For this review, take the finished solid that the model builds, in its own axes (mm). Face numbers are marked on the shaded views. A direction names the side the tool comes from. Give positions to 0.01 mm unless a question says otherwise; leave off trailing zeros. Order: outer loops, then holes, each group sorted by start corner. A loop starts at its lowest first (then second) coordinate and runs counter-clockwise, first axis right, second up.
Item 1: The part is to be moulded in two halves that separate along X. For the marked faces 4, 5 and 6, say which applies: released by +X, released by -X, zero draft, split by the parting line, or undercut.
Item 2: For probe 1 along X at (y, z) = (1.75, -10.75); probe 2 along X at (y, z) = (8.5, -14.25); probe 3 along Y at (x, z) = (-4, -9), list the stretches that pass through material, from the lowest coordinate up.
Item 3: Consider section A-A (x = 0). Give the boundary of the cut face in (y, z), plus the area to 3 significant figures.
Item 4: Consider section D-D (x = 2.5). Give the boundary of the cut face in (y, z), plus the area to 3 significant figures.
Item 5: Machinability: for the marked faces 1, 2 and 3, which of the approach directions +Z, -Z, +X, -X, +Y, -Y give a long, thin tool a straight path to every point of the face, cutting with its end or side? Answer none if there is none.
Item 6: Consider section B-B (z = -11). Give the boundary of the cut face in (x, y), plus the area to 3 significant figures.
Item 7: For P1, Ø6, axis at y = 16, z = -10.5, coming from the -X side; P2, Ø1, axis at x = 4, z = -17.5, coming from the +Y side, all flat-tipped, find the tip position at first contact; note any pin that passes through.
Item 8: Consider section C-C (y = 12). Give the boundary of the cut face in (x, z), plus the area to 3 significant figures.
```python
from build123d import *

# Parameters (mm, degrees)
BODY_DEPTH     = 8.5
SKETCH2_W      = 13
SKETCH2_H      = 17
EXTUSION_DEPTH = 18
HOLE_A_DEPTH   = 29.217902119
HOLE_B_DEPTH   = 17


with BuildPart() as part:
    # Sketch1 → Body (new, symmetric)
    with BuildSketch(Plane(origin=(0, 0, 0), x_dir=(0, 0, -1), z_dir=(1, 0, 0))):
        Polygon((3, 20), (0, 20), (0, 0), (20, 0), (20, 3), align=None)
    extrude(amount=BODY_DEPTH, both=True)

    # Sketch2 → Extusion (cut)
    with BuildSketch(Plane(origin=(0, 0, -20), x_dir=(-1, 0, 0), z_dir=(0, 0, -1))):
        with Locations((0, 11.5)):
            Rectangle(SKETCH2_W, SKETCH2_H)
    extrude(amount=-EXTUSION_DEPTH, mode=Mode.SUBTRACT)

    # Sketch3 → Hole_A (cut, through all)
    with BuildSketch(Plane(origin=(0, 0, -2), x_dir=(-1, 0, 0), z_dir=(0, 0, -1))):
        with BuildLine():
            Line((-3.25, 7.5), (-3.25, 12.5))
            ThreePointArc((-3.25, 12.5), (0, 15.75), (3.25, 12.5))
            Line((3.25, 12.5), (3.25, 7.5))
            ThreePointArc((3.25, 7.5), (0, 4.25), (-3.25, 7.5))
        make_face()
    extrude(amount=-HOLE_A_DEPTH, mode=Mode.SUBTRACT)

    # Sketch4 → Hole_B (cut)
    with BuildSketch(Plane(origin=(0, 3, 0), x_dir=(1, 0, 0), z_dir=(0, 1, 0))):
        with BuildLine():
            Line((-3.25, 7.5), (-3.25, 12.5))
            ThreePointArc((-3.25, 12.5), (0, 15.75), (3.25, 12.5))
            Line((3.25, 12.5), (3.25, 7.5))
            ThreePointArc((3.25, 7.5), (0, 4.25), (-3.25, 7.5))
        make_face()
    extrude(amount=-HOLE_B_DEPTH, mode=Mode.SUBTRACT)


solid = part.part
```
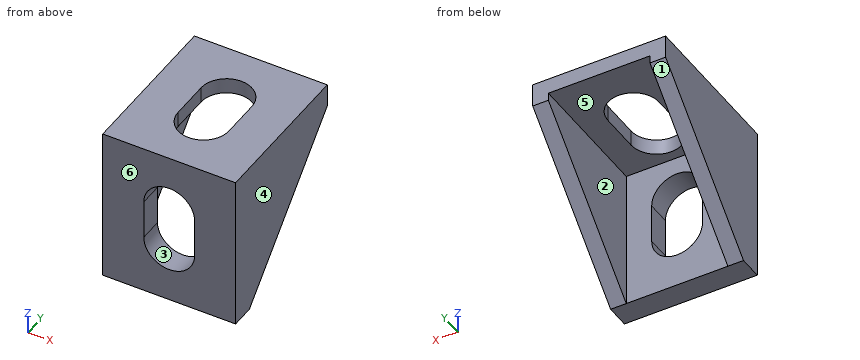
Resolved:
1. face 4: released by +X
1. face 5: undercut
1. face 6: zero draft
2. probe 1: x = -8.5 to -3.25, 3.25 to 8.5
2. probe 2: x = -8.5 to -6.5, 6.5 to 8.5
2. probe 3: y = 0 to 3
3. outline: (0, -20) - (3, -20) - (3, -15.75) - (0, -15.75) - close; (0, -4.25) - (3, -4.25) - (3, -2) - (4.25, -2) - (4.25, 0) - (0, 0) - close; (15.75, -2) - (20, -2) - (20, 0) - (15.75, 0) - close
3. area: 36.5 mm2
4. outline: (0, -20) - (3, -20) - (3, -14.58) - (0, -14.58) - close; (0, -5.42) - (3, -5.42) - (3, -2) - (5.42, -2) - (5.42, 0) - (0, 0) - close; (14.58, -2) - (20, -2) - (20, 0) - (14.58, 0) - close
4. area: 48.2 mm2
5. face 1: -Z, +X, -X, +Y
5. face 2: -Z, +Y
5. face 3: +Y, -Y
6. outline: (-8.5, 0) - (-3.25, 0) - (-3.25, 3) - (-6.5, 3) - (-6.5, 12) - (-8.5, 12) - close; (3.25, 0) - (8.5, 0) - (8.5, 12) - (6.5, 12) - (6.5, 3) - (3.25, 3) - close
6. area: 67.5 mm2
7. P1: stops at x = -8.5
7. P2: stops at y = 3
8. outline: (-8.5, -11) - (-6.5, -11) - (-6.5, -2) - (-3.25, -2) - (-3.25, 0) - (-8.5, 0) - close; (3.25, -2) - (6.5, -2) - (6.5, -11) - (8.5, -11) - (8.5, 0) - (3.25, 0) - close
8. area: 57.0 mm2
